Check sheet for the drawn part. Datum: minimum x, y, z corner. Units: mm. A direction names the side the tool comes from. Coordinates: 2 decimals unless noted, no trailing zeros. Loops run counter-clockwise (first coordinate to the right, second up) from the corner with the lowest first, then second, coordinate; pieces in that order, holes last.
Q1. Sectioned sample at C-C (z = 3.4). Enter the section's corners in (x, y).
Q2. Access from +Z, -Z, +X, -X, +Y, -Y to the whole of each face (thin tool, end or side, straight path). Record for the marked faces 1, 2 and 3.
Q3. Sectioned sample at A-A (x = 18). Enter the section's corners in (y, z).
Q4. Sectioned sample at D-D (x = 1.5). Enter the section's corners in (y, z), then the cut area to 3 significant figures.
Q5. Sectioned sample at B-B (z = 2). Enter the section's corners in (x, y), then the cut area to 3 significant figures.
Q6. Material ranges on probe 1 along X at (y, z) = (0.9, 2); probe 2 along Y at (x, z) = (12, 1.1); probe 3 along X at (y, z) = (22.5, 3.45), recorded low to high.
Q7. Go/stop test with flat-tipped pins: P1, Ø6, axis at x = 17, y = 20, coming from the +Z side; P2, Ø2, axis at x = 10, z = 2, coming from the +Y side; P3, Ø2, axis at y = 9.5, z = 2, coming from the +X side; P4, Ø2, axis at y = 5.5, z = 2.5, coming from the -X side. Record where each tip stops, or that it passes through.
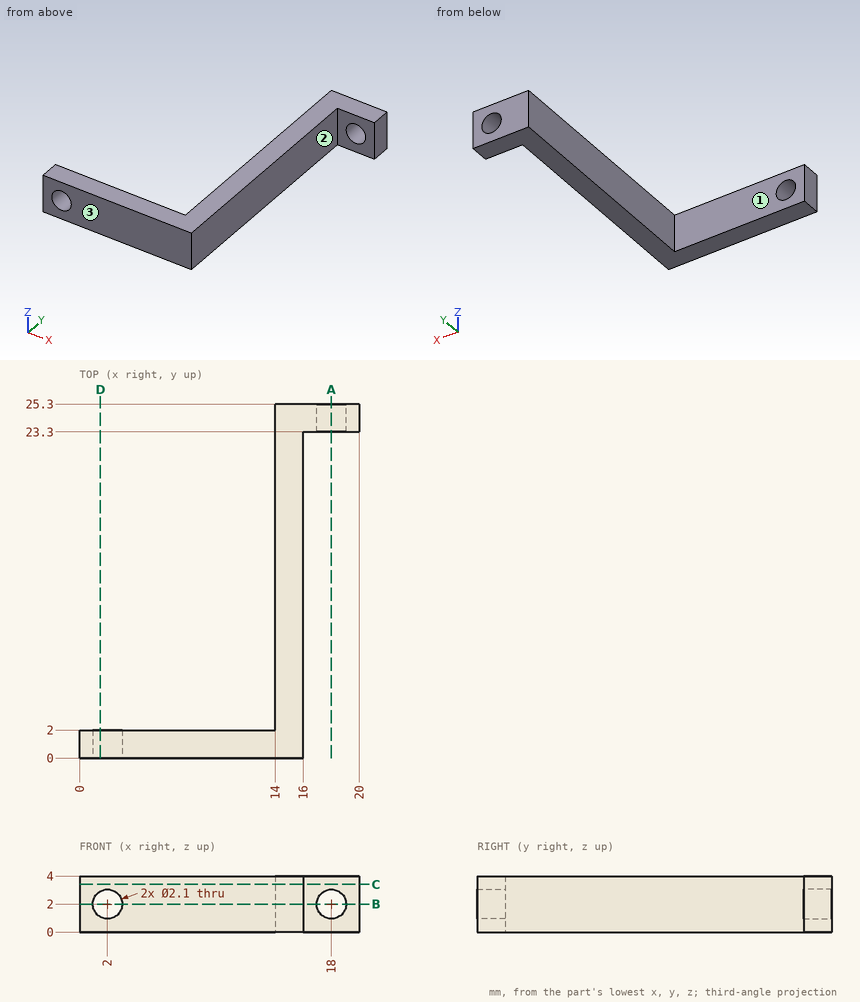
Geometry check:
1. outline: (0, 0) - (16, 0) - (16, 23.3) - (20, 23.3) - (20, 25.3) - (14, 25.3) - (14, 2) - (0, 2) - close
2. face 1: +Z, -Z, -X, +Y
2. face 2: +Z, -Z, +X, -Y
2. face 3: +Z, -Z, +X, -X, -Y
3. outline: (23.3, 0) - (25.3, 0) - (25.3, 0.95) - (23.3, 0.95) - close; (23.3, 3.05) - (25.3, 3.05) - (25.3, 4) - (23.3, 4) - close
4. outline: (0, 0) - (2, 0) - (2, 1.08) - (0, 1.08) - close; (0, 2.92) - (2, 2.92) - (2, 4) - (0, 4) - close
4. area: 4.31 mm2
5. outline: (0, 0) - (0.95, 0) - (0.95, 2) - (0, 2) - close; (3.05, 0) - (16, 0) - (16, 23.3) - (16.95, 23.3) - (16.95, 25.3) - (14, 25.3) - (14, 2) - (3.05, 2) - close; (19.05, 23.3) - (20, 23.3) - (20, 25.3) - (19.05, 25.3) - close
5. area: 78.2 mm2
6. probe 1: x = 0 to 0.95, 3.05 to 16
6. probe 2: y = 0 to 2
6. probe 3: x = 14 to 16
7. P1: stops at z = 4
7. P2: stops at y = 2
7. P3: stops at x = 16
7. P4: stops at x = 14
